Autodesk Inventor part; units mm, degrees
ref_plane "YZ Plane" through (0, 0, 0) normal (1, 0, 0) x (0, 1, 0)
ref_plane "XZ Plane" through (0, 0, 0) normal (0, 1, 0) x (-1, 0, 0)
ref_plane "XY Plane" through (0, 0, 0) normal (0, 0, 1) x (1, 0, 0)
sketch "Sketch1" plane through (0, 0, 0) normal (0, 1, 0) x (-1, 0, 0)
  line L0 (0, 0) -> (-89, 0)
  line L1 (-89, 0) -> (-89, 84)
  line L2 (-89, 84) -> (0, 84)
  line L3 (0, 84) -> (0, 0)
  dimension "d0" = 89
  dimension "d1" = 84
extrude "Extrusion1" add sketch "Sketch1" along normal blind 14
fillet "Fillet1" radius 2 4 edges at (44.5, 14, 0) (0, 14, 42) (89, 14, 42) (44.5, 14, 84)
sketch "Sketch2" plane through (0, 14, 0) normal (0, 1, 0) x (1, 0, 0)
  line L0 (89, 0) -> (0, 0)
  line L1 (6.9319, 0) -> (15.3203, 0)
  line L2 (15.3203, 0) -> (15.3203, -11.7863)
  line L3 (15.3203, -11.7863) -> (6.9319, -11.7863)
  line L4 (6.9319, -11.7863) -> (6.9319, 0)
  line L5 (20.9884, 0) -> (29.3768, 0)
  line L6 (29.3768, 0) -> (29.3768, -11.7863)
  line L7 (29.3768, -11.7863) -> (20.9884, -11.7863)
  line L8 (20.9884, -11.7863) -> (20.9884, 0)
  line L9 (67.6628, 0) -> (76.0512, 0)
  line L10 (76.0512, 0) -> (76.0512, -11.7863)
  line L11 (76.0512, -11.7863) -> (67.6628, -11.7863)
  line L12 (67.6628, -11.7863) -> (67.6628, 0)
  line L13 (7, -84.0181) -> (15.3884, -84.0181)
  line L14 (15.3884, -84.0181) -> (15.3884, -72.2317)
  line L15 (15.3884, -72.2317) -> (7, -72.2317)
  line L16 (7, -72.2317) -> (7, -84.0181)
  line L17 (89, -84) -> (0, -84)
extrude "Extrusion2" cut sketch "Sketch2" against normal blind 5
properties part number "RomeoSudoController"
The listing builds one solid part. Answer for the finished solid, in the listing's coordinates (mm). A direction names the side the tool comes from. Round coordinates to 2 decimals unless told otherwise and drop trailing zeros. Loops run counter-clockwise (first coordinate to the right, second up) from the corner with the lowest first, then second, coordinate; pieces in that order, holes last. Notation, with made-up numbers: M -4,-12 L 36,-12 A23 ccw 36,21 Z; hole C 48,14.5 d2. An arc over 180 degrees is marked long. Return JSON: item names as keys, results as strings.
Q1. Each of these flat-tipped pins is pushed along its axis until it touches: pin 1 Ø4 at (x, z) = (11.5, 78) entering from +Y; pin 2 Ø4 at (x, y) = (9, 12.5) entering from -Z; pin 3 Ø5.5 at (x, y) = (11.5, 12) entering from +Z. Where does it stop, or does it pass through?
Results list:
{"pin 1": "stops at y = 9", "pin 2": "stops at z = 11.79", "pin 3": "stops at z = 72.23"}
Q2. Which of the six approach directions +Z, -Z, +X, -X, +Y, -Y give full straight-line access (tool end or side, diameter ignored) to faces 1 (the face through (45, 14, 43)), 2 (the face through (6.932, 12, 6)), 3 (the face through (11, 9, 78))?
Results list:
{"face 1": "+Z, -Z, +X, -X, +Y", "face 2": "-Z, +Y", "face 3": "+Z, +Y"}
Q3. Find the intervals of material crossed by line 1 along Y through (x, z) = (22.5, 6); line 2 along Z through (x, y) = (29, 11.75); line 3 along Z through (x, y) = (12, 13), in increasing order. Write a range as from..to.
Results list:
{"line 1": "y = 0..9", "line 2": "z = 11.79..84", "line 3": "z = 11.79..72.23"}
Q4. Find section B-B, the plane x = 24. Determine the outline of the cut face in (y, z), plus the area to 3 significant figures.
Results list:
{"outline": "M 0,0 L 9,0 L 9,11.79 L 14,11.79 L 14,82 A2 ccw 12,84 L 0,84 Z", "area": "1,120 mm2"}
Q5. Find section A-A, the plane z = 9. Determine the outline of the cut face in (x, y).
Results list:
{"outline": "M 0,0 L 89,0 L 89,12 A2 ccw 87,14 L 76.05,14 L 76.05,9 L 67.66,9 L 67.66,14 L 29.38,14 L 29.38,9 L 20.99,9 L 20.99,14 L 15.32,14 L 15.32,9 L 6.93,9 L 6.93,14 L 2,14 A2 ccw 0,12 Z"}
Q6. The mould has two halves that part along X. Classify faces 4 (the face through (7, 12, 78)), 5 (the face through (89, 6, 41)), 6 (the face through (45, 0, 43)), 7 (the face through (0, 6, 43)): released by +X, released by -X, zero draft, split by the parting line, or undercut.
Results list:
{"face 4": "undercut", "face 5": "released by +X", "face 6": "zero draft", "face 7": "released by -X"}
Q7. Find section C-C, the plane z = 74.5. Determine the outline of the cut face in (x, y).
Results list:
{"outline": "M 0,0 L 89,0 L 89,12 A2 ccw 87,14 L 15.39,14 L 15.39,9 L 7,9 L 7,14 L 2,14 A2 ccw 0,12 Z"}
